Could you check a few things on this model? Use its own coordinates, in mm. Face numbers are marked on the shaded views. Coordinates: 2 decimals unless noted, no trailing zeros. Loops run counter-clockwise (first coordinate to the right, second up) from the corner with the lowest first, then second, coordinate; pieces in that order, holes last.
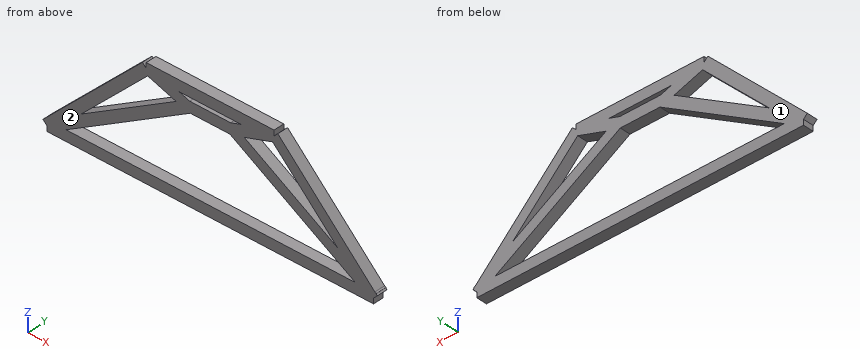
from build123d import *

# Parameters (mm, degrees)
F8_W      = 584.2
F8_H      = 19.05
F4_W      = 76.2
F4_H      = 19.05
F2_W      = 228.6
F2_H      = 19.05
F10_DEPTH = 19.05


with BuildPart() as f10:
    # F5 (on Front) + F8 (on Front) + F6 (on Front) + F7 (on Front) + F9 (on Front) + F4 (on Front) + F1 (on Front) + F2 (on Front) + F3 (on Front) → F10 (new body)
    with BuildSketch(Plane.XZ):
        Polygon((-93.580917, 161.435332), (-87.556597, 143.362975), (-11.356597, 168.763822), (-17.380917, 186.836178), align=None)
    with BuildSketch(Plane.XZ):
        with Locations((-128.666217, 0)):
            Rectangle(F8_W, F8_H)
    with BuildSketch(Plane.XZ):
        Polygon((-425.666789, 8.16762), (-415.865645, -8.16762), (-161.865645, 144.23238), (-171.666789, 160.56762), align=None)
    with BuildSketch(Plane.XZ):
        Polygon((-21.101361, 171.06222), (156.698639, -6.73524), (170.168927, 6.73524), (-7.631073, 184.5327), align=None)
    with BuildSketch(Plane.XZ):
        Polygon((-85.698658, 160.587338), (-95.433776, 144.212662), (158.566224, -6.796122), (168.301342, 9.578553), align=None)
    with BuildSketch(Plane.XZ):
        with Locations((-128.666217, 152.4)):
            Rectangle(F4_W, F4_H)
    with BuildSketch(Plane.XZ):
        Polygon((-249.703997, 184.535144), (-427.501457, 6.735144), (-414.030977, -6.735144), (-236.233517, 171.064856), align=None)
    with BuildSketch(Plane.XZ):
        with Locations((-128.668757, 177.8)):
            Rectangle(F2_W, F2_H)
    with BuildSketch(Plane.XZ):
        Polygon((-239.645784, 186.732577), (-246.29173, 168.867423), (-170.08665, 143.466576), (-163.445784, 161.333424), align=None)
    extrude(amount=F10_DEPTH)


solid = f10.part
(1) I need wall thicknesses on probe 1 along Z at (x, y) = (-127, -14.5) (3 decimals); probe 2 along X at (y, z) = (-12.5, 118); probe 3 along Z at (x, y) = (8.5, -1) (3 decimals). Which ranges of each line are inside material? Lowest first, please.
Answers:
probe 1: z = -9.525 to 9.525, 142.875 to 161.925, 168.275 to 187.325
probe 2: x = -316.24 to -289.3, -242.61 to -205.59, -51.34 to -14.07, 31.96 to 58.9
probe 3: z = -9.525 to 9.525, 82.422 to 104.584, 141.461 to 168.402
(2) Imagine slicing it at B-B, the plane z = 22.5. Write out the boundary of the cut face in (x, y).
Answers:
outline: (-411.74, -19.05) - (-364.75, -19.05) - (-364.75, 0) - (-411.74, 0) - close; (109.29, -19.05) - (154.4, -19.05) - (154.4, 0) - (109.29, 0) - close
(3) Imagine slicing it at D-D, the plane x = -372. Write out the boundary of the cut face in (y, z) (3 decimals), and give its area (3 significant figures).
Answers:
outline: (-19.05, -9.525) - (0, -9.525) - (0, 9.525) - (-19.05, 9.525) - close; (-19.05, 18.152) - (0, 18.152) - (0, 62.237) - (-19.05, 62.237) - close
area: 1,200 mm2
(4) For pin 1 (6 mm diameter, centred on y = -13, z = 137.5, fed in from -X); pin 2 (6 mm diameter, centred on y = -13.5, z = 90, fed in from +X); pin 3 (8 mm diameter, centred on x = -353, y = -14.5, fed in from +Z), each with a flat end and sliding along its axis, tell me the tip position at first contact or that it passes through.
Answers:
pin 1: stops at x = -299.74
pin 2: stops at x = 89.9
pin 3: stops at z = 85.24
(5) Imagine slicing it at A-A, the plane y = -12.5. State how many separate pieces and enclosed holes the cut face has, and give its area (3 significant figures).
Answers:
separate pieces: 1
enclosed holes: 4
area: 37,000 mm2
(6) We'd pull the mould along Y, two halves only. Please class the marked faces 1 and 2: +Y half, -Y half, draft (parallel to the pull), parting line (faces both ways), or undercut.
Answers:
face 1: +Y half
face 2: -Y half
(7) Imagine slicing it at C-C, the plane x = -195.5. Write out the boundary of the cut face in (y, z) (3 decimals), and give its area (3 significant figures).
Answers:
outline: (-19.05, -9.525) - (0, -9.525) - (0, 9.525) - (-19.05, 9.525) - close; (-19.05, 124.052) - (0, 124.052) - (0, 146.268) - (-19.05, 146.268) - close; (-19.05, 151.937) - (0, 151.937) - (0, 187.325) - (-19.05, 187.325) - close
area: 1,460 mm2
